Autodesk Inventor part; units mm, degrees
ref_plane "YZ Plane" through (0, 0, 0) normal (1, 0, 0) x (0, 1, 0)
ref_plane "XZ Plane" through (0, 0, 0) normal (0, 1, 0) x (-1, 0, 0)
ref_plane "XY Plane" through (0, 0, 0) normal (0, 0, 1) x (1, 0, 0)
sketch "スケッチ1" plane through (0, 0, 0) normal (0, 0, 1) x (1, 0, 0)
  circle A0 centre (0, 0) radius 12
  circle A1 centre (0, 8.5) radius 1.35
  circle A2 centre (0, 0) radius 1.2
  circle A3 centre (-8.5, 0) radius 1.35
  circle A4 centre (0, -8.5) radius 1.35
  circle A5 centre (8.5, 0) radius 1.35
  dimension "d0" = 2.7
  dimension "d1" = 8.5
  dimension "d2" = 24
  dimension "d3" = 2.4
  dimension "d6" = 360
extrude "押し出し1" add sketch "スケッチ1" along normal blind 1.5
sketch "スケッチ2" plane through (0, 0, 1.5) normal (0, 0, 1) x (1, 0, 0)
  circle A0 centre (0, 0) radius 1.2
  circle A1 centre (0, 0) radius 12
  circle A2 centre (0, 0) radius 2.45
  dimension "d10" = 4.9
extrude "押し出し2" add sketch "スケッチ2" along normal blind 3.5 contours A2
sketch "スケッチ3" plane through (0, 0, 1.5) normal (0, 0, 1) x (1, 0, 0)
  circle A0 centre (0, 0) radius 2.45
  circle A1 centre (0, 8.5) radius 1.35
  point P0 (-8.5, 0)
  point P1 (0, -8.5)
  point P2 (8.5, 0)
  dimension "d15" = 360
hole "穴1" at (0, 8.5, 1.5) at (-8.5, 0, 1.5) at (0, -8.5, 1.5) at (8.5, 0, 1.5) direction (0, 0, -1) diameter 5 depth 1
properties part number "足首_独立ピッチ_1_2" material "アルミニウム 2014-T4"
Work out the finished part from the listing and answer in its coordinate system (mm). A direction names the side the tool comes from. Give positions to 0.01 mm unless a question says otherwise; leave off trailing zeros. Order: outer loops, then holes, each group sorted by start corner. A loop starts at its lowest first (then second) coordinate and runs counter-clockwise, first axis right, second up. Notation, with made-up numbers: (41.25, 14.5) -> (85.25, 14.5) arc R12 ccw to (85.25, 30.5) -> close; hole circle Ø3 at (81, 60.25). An arc over 180 degrees is marked (long way). Answer as a JSON object with one key per item and string values. Group by question number.
1. Consider line 1 along Y through (x, z) = (0, 0.95); line 2 along Y through (x, z) = (-0.75, 1.05); line 3 along Y through (x, z) = (2, 1.3). Determine where each line is inside the solid, lowest interval first. Write a range as [from, to].
2. Section C-C on z = 3.6 is taken. Determine the outline of the cut face in (x, y), plus the area to 3 significant figures.
3. Section B-B on y = 8.5 is taken. Determine the outline of the cut face in (x, z), plus the area to 3 significant figures.
4. Flat-ended cylindrical pins translate along their axes: pin 1 Ø2 at (x, y) = (3.5, -4) entering from +Z; pin 2 Ø2 at (x, z) = (2.5, 3.5) entering from +Y; pin 3 Ø3 at (x, y) = (-8.5, 0) entering from +Z. Find the tip coordinate at first contact, or state that the pin passes through.
5. Section A-A on x = 0 is taken. Determine the outline of the cut face in (y, z), plus the area to 4 significant figures.
6. A tool of negligible diameter and unlimited length cuts with its end or side. For faces 4 (the flat face through (-7, -1, 0.5)), 5 (the cylindrical face through (0.65, -1.01, 2.46)), from which of +Z, -Z, +X, -X, +Y, -Y can it reach the whole face along a straight path? Write none if from no direction.
7. The mould has two halves that part along X. Classify faces 1 (the flat face through (0, 3, 1.5)), 2 (the cylindrical face through (-11.99, -0.53, 0.74)), 3 (the cylindrical face through (9.788, -0.406, 0.246)): released by +X, released by -X, zero draft, split by the parting line, or undercut.
Result sheet:
{
 "1": {"line 1": "y = [-12, -11], [-6, -1.2], [1.2, 6], [11, 12]", "line 2": "y = [-11.98, -10.88], [-6.12, -0.94], [0.94, 6.12], [10.88, 11.98]", "line 3": "y = [-11.83, -10], [-7, 7], [10, 11.83]"},
 "2": {"outline": "circle Ø4.9 at (0, 0); hole circle Ø2.4 at (0, 0)", "area": "14.3 mm^2"},
 "3": {"outline": "(-8.47, 0) -> (-1.35, 0) -> (-1.35, 0.5) -> (-2.5, 0.5) -> (-2.5, 1.5) -> (-8.47, 1.5) -> close; (1.35, 0) -> (8.47, 0) -> (8.47, 1.5) -> (2.5, 1.5) -> (2.5, 0.5) -> (1.35, 0.5) -> close", "area": "19.1 mm^2"},
 "4": {"pin 1": "stops at z = 1.5", "pin 2": "stops at y = 1.94", "pin 3": "stops at z = 0.5"},
 "5": {"outline": "(-12, 0) -> (-9.85, 0) -> (-9.85, 0.5) -> (-11, 0.5) -> (-11, 1.5) -> (-12, 1.5) -> close; (-7.15, 0) -> (-1.2, 0) -> (-1.2, 5) -> (-2.45, 5) -> (-2.45, 1.5) -> (-6, 1.5) -> (-6, 0.5) -> (-7.15, 0.5) -> close; (1.2, 0) -> (7.15, 0) -> (7.15, 0.5) -> (6, 0.5) -> (6, 1.5) -> (2.45, 1.5) -> (2.45, 5) -> (1.2, 5) -> close; (9.85, 0) -> (12, 0) -> (12, 1.5) -> (11, 1.5) -> (11, 0.5) -> (9.85, 0.5) -> close", "area": "28.45 mm^2"},
 "6": {"face 4": "+Z", "face 5": "+Z, -Z"},
 "7": {"face 1": "zero draft", "face 2": "split by the parting line", "face 3": "undercut"}
}
